The listing builds one solid part. Answer for the finished solid, in the listing's coordinates (mm). A direction names the side the tool comes from. Round coordinates to 2 decimals unless told otherwise and drop trailing zeros. Order: outer loops, then holes, each group sorted by start corner. A loop starts at its lowest first (then second) coordinate and runs counter-clockwise, first axis right, second up. Notation, with made-up numbers: M 19.5,-18 L 64.5,-18 A21 cw 64.5,7 Z; hole C 63,19.25 d2. An arc over 180 degrees is marked long. Write item = value, one per line. Start each with the question number.
(1) A cutting plane is placed at D-D, the plane y = -18.5. Determine the outline of the cut face in (x, z) (3 decimals).
(2) A cutting plane is placed at A-A, the plane x = 26. Determine the outline of the cut face in (y, z) (3 decimals), and give its area (3 significant figures).
(3) Which of the six approach directions +Z, -Z, +X, -X, +Y, -Y give full straight-line access (tool end or side, diameter ignored) to faces 5 (the face through (22.105, -33.49, 30.051)), 6 (the face through (29.67, -24.166, 22.136)), 7 (the face through (13, -30.468, 20))?
(4) A cutting plane is placed at B-B, the plane z = 8. Determine the outline of the cut face in (x, y), and give its area (3 significant figures).
(5) A cutting plane is placed at C-C, the plane y = -29. Determine the outline of the cut face in (x, z) (3 decimals).
(6) Each of these flat-tipped pins is pushed along its axis until it touches: pin 1 (2 mm diameter, centred on y = -24, z = 23, fed in from -X); pin 2 (2.5 mm diameter, centred on x = 25, y = -19.5, fed in from +Z) (3 decimals); pin 3 (9.5 mm diameter, centred on x = 12.5, z = 14.5, fed in from -Y); pin 4 (8 mm diameter, centred on y = -12, z = 32, fed in from +X). Where does it stop, or does it pass through?
(7) For a pull along X with two mould halves and no side action, classify faces 1 (the face through (22.105, -4.71, 30.051)), 2 (the face through (25.4, -30, 23)), 3 (the face through (13.44, -5.84, 17.2)), 4 (the face through (29.345, -29.246, 27.143)) as released by +X, released by -X, zero draft, split by the parting line, or undercut.
(8) Straight lines are drawn through the part: probe 1 along Y at (x, z) = (2.5, 9.5); probe 2 along Y at (x, z) = (22, 25.5); probe 3 along X at (y, z) = (-3.5, 25). For each, find the intervals that lie inside material, in ascending order. Write a range as from..to.
from build123d import *

# Parameters (mm, degrees)
F0_W      = 37.9036115915
F0_H      = 38.1
F1_DEPTH  = 38.1
F6_DEPTH  = 38.1
F8_DEPTH  = 38.1
F9_W      = 25.4
F9_H      = 7.62
F10_DEPTH = 38.1


# Not quite as in the source:
# - a feature names something its author has since deleted; it is built from what else it names


with BuildPart() as f1:
    # F0 (on Front) → F1 (new body)
    with BuildSketch(Plane.XZ):
        with Locations((18.9518057957, 19.05)):
            Rectangle(F0_W, F0_H)
    extrude(amount=F1_DEPTH)

    # F5 (on offset) → F6 (cut)
    with BuildSketch(Plane.YZ.offset(38.1)):
        Polygon((-6.35, 38.1), (-31.75, 38.1), (-26.67, 15.875), (-21.59, 28.575), (-16.51, 28.575), (-11.43, 15.875), align=None)
        Polygon((-31.75, 0), (-38.1, 38.1), (-38.1, 0), align=None)
        Polygon((-19.5393956542, 15.875), (-25.4, 0), (-12.7, 0), align=None)
        Polygon((0, 0), (0, 38.1), (-6.35, 0), align=None)
    extrude(amount=-F6_DEPTH, mode=Mode.SUBTRACT)

    # F7 (on offset) → F8 (cut)
    with BuildSketch(Plane.XZ.offset(38.1)):
        Polygon((25.2844232855, 38.196389037), (12.7511301009, 38.2289945719), (19.05, 22.225), align=None)
        Polygon((11.43, 22.225), (6.35, 0), (31.75, 0), (26.67, 22.225), (21.589256481, 9.4380885469), (16.51, 9.525), align=None)
        Polygon((38.1, 38.1630491376), (31.7472500896, 38.179575904), (31.75, 38.1630491376), (38.1, 0), align=None)
        Polygon((6.35, 38.2456472001), (0, 38.2621668126), (0, 0), align=None)
    extrude(amount=-F8_DEPTH, mode=Mode.SUBTRACT)

    # F9 (on offset) → F10 (cut)
    with BuildSketch(Plane.XY.offset(38.1)):
        with Locations((25.4, -11.43)):
            Rectangle(F9_W, F9_H)
        with Locations((12.7, -26.6583908668)):
            Rectangle(F9_W, F9_H)
    extrude(amount=-F10_DEPTH, mode=Mode.SUBTRACT)


solid = f1.part
Reported:
q1.outline = M 2.235,13.462 L 9.427,13.462 L 11.43,22.225 L 14.935,13.462 L 23.188,13.462 L 26.67,22.225 L 28.673,13.462 L 35.86,13.462 L 33.345,28.575 L 21.529,28.575 L 19.05,22.225 L 16.551,28.575 L 4.744,28.575 Z
q2.outline = M -38.1,38.1 L -35.173,20.539 L -27.736,20.539 L -31.75,38.1 Z; M -24.804,20.539 L -15.24,20.539 L -15.24,25.4 L -16.51,28.575 L -21.59,28.575 Z; M -7.62,20.539 L -2.927,20.539 L 0,38.1 L -6.35,38.1 L -7.62,32.544 Z
q2.area = 288 mm²
q3.face_5 = +Z, +Y, -Y
q3.face_6 = +Z, +X, -X
q3.face_7 = +Z, -Z, -X
q4.outline = M 1.33,-33.08 L 8.18,-33.08 L 8.18,-30.47 L 1.33,-30.47 Z; M 1.33,-22.85 L 8.18,-22.85 L 8.18,-22.45 L 1.33,-22.45 Z; M 1.33,-16.15 L 8.18,-16.15 L 8.18,-5.02 L 1.33,-5.02 Z; M 29.92,-33.08 L 36.77,-33.08 L 36.77,-22.45 L 29.92,-22.45 Z; M 29.92,-16.15 L 36.77,-16.15 L 36.77,-15.24 L 29.92,-15.24 Z; M 29.92,-7.62 L 36.77,-7.62 L 36.77,-5.02 L 29.92,-5.02 Z
q4.area = 194 mm²
q5.outline = M 25.4,19.029 L 26.67,22.225 L 31.75,0 L 37.904,0 L 37.904,1.18 L 33.762,26.069 L 25.4,26.069 Z
q6.pin_1 = 25.4
q6.pin_2 = 28.575
q6.pin_3 = -34.96
q6.pin_4 = through
q7.face_1 = undercut
q7.face_2 = released by -X
q7.face_3 = undercut
q7.face_4 = zero draft
q8.probe_1 = -33.33..-30.47, -22.85..-21.89, -16.79..-4.77
q8.probe_2 = -36..-30.47, -22.82..-15.28, -7.62..-2.1
q8.probe_3 = 4.15..17.96, 20.13..33.94
